Autodesk Inventor part; units mm, degrees
ref_plane "YZ Plane" through (0, 0, 0) normal (1, 0, 0) x (0, 1, 0)
ref_plane "XZ Plane" through (0, 0, 0) normal (0, 1, 0) x (-1, 0, 0)
ref_plane "XY Plane" through (0, 0, 0) normal (0, 0, 1) x (1, 0, 0)
sketch "Sketch1" plane through (0, 0, 0) normal (0, 0, 1) x (1, 0, 0)
  line L0 (0, 0) -> (190, 0)
  line L1 (0, 140) -> (0, 0)
  line L2 (190, 0) -> (190, 30)
  line L3 (190, 30) -> (210, 30)
  line L4 (210, 30) -> (210, 74.5)
  line L5 (186, 140) -> (186, 74.5)
  line L6 (186, 74.5) -> (210, 74.5)
  line L7 (186, 140) -> (0, 140)
  dimension "d2" = 20
  dimension "d3" = 30
  dimension "d4" = 140
  dimension "d49" = 24
  dimension "d50" = 65.5
  dimension "d51" = 210
extrude "Extrusion1" add sketch "Sketch1" along normal blind 3
sketch "Sketch2" plane through (0, 0, 3) normal (0, 0, 1) x (1, 0, 0)
  arc A0 (141.1, 85.2251) -> (158.9, 85.2251) centre (150, 90) ccw
  line L0 (210, 30) -> (210, 74.5)
  line L1 (250, 140) -> (0, 140)
  line L2 (141.1, 94.7749) -> (141.1, 85.2251)
  line L3 (158.9, 94.7749) -> (158.9, 85.2251)
  arc A1 (158.9, 94.7749) -> (141.1, 94.7749) centre (150, 90) ccw
  circle A2 centre (180, 114) radius 6
  line L4 (158.9, 54.7749) -> (158.9, 45.2251)
  arc A3 (158.9, 54.7749) -> (141.1, 54.7749) centre (150, 50) ccw
  line L5 (141.1, 54.7749) -> (141.1, 45.2251)
  arc A4 (141.1, 45.2251) -> (158.9, 45.2251) centre (150, 50) ccw
  arc A5 (101.1, 85.2251) -> (118.9, 85.2251) centre (110, 90) ccw
  arc A6 (118.9, 94.7749) -> (101.1, 94.7749) centre (110, 90) ccw
  line L6 (118.9, 94.7749) -> (118.9, 85.2251)
  line L7 (101.1, 94.7749) -> (101.1, 85.2251)
  arc A7 (63.25, 96.4) -> (76.75, 96.4) centre (70, 100) ccw
  line L8 (63.25, 103.6) -> (63.25, 96.4)
  line L9 (76.75, 103.6) -> (76.75, 96.4)
  arc A8 (76.75, 103.6) -> (63.25, 103.6) centre (70, 100) ccw
  line L10 (76.75, 73.6) -> (76.75, 66.4)
  arc A9 (63.25, 66.4) -> (76.75, 66.4) centre (70, 70) ccw
  line L11 (63.25, 73.6) -> (63.25, 66.4)
  arc A10 (76.75, 73.6) -> (63.25, 73.6) centre (70, 70) ccw
  line L12 (76.75, 43.6) -> (76.75, 36.4)
  arc A11 (63.25, 36.4) -> (76.75, 36.4) centre (70, 40) ccw
  line L13 (63.25, 43.6) -> (63.25, 36.4)
  arc A12 (76.75, 43.6) -> (63.25, 43.6) centre (70, 40) ccw
  line L14 (36.75, 103.6) -> (36.75, 96.4)
  arc A13 (23.25, 96.4) -> (36.75, 96.4) centre (30, 100) ccw
  line L15 (23.25, 103.6) -> (23.25, 96.4)
  arc A14 (36.75, 103.6) -> (23.25, 103.6) centre (30, 100) ccw
  line L16 (36.75, 73.6) -> (36.75, 66.4)
  arc A15 (23.25, 66.4) -> (36.75, 66.4) centre (30, 70) ccw
  line L17 (23.25, 73.6) -> (23.25, 66.4)
  arc A16 (36.75, 73.6) -> (23.25, 73.6) centre (30, 70) ccw
  line L18 (36.75, 43.6) -> (36.75, 36.4)
  arc A17 (23.25, 36.4) -> (36.75, 36.4) centre (30, 40) ccw
  line L19 (23.25, 43.6) -> (23.25, 36.4)
  arc A18 (36.75, 43.6) -> (23.25, 43.6) centre (30, 40) ccw
  circle A19 centre (180, 99) radius 6
  circle A20 centre (180, 84) radius 6
  circle A21 centre (180, 69) radius 6
  point P0 (0, 0)
  dimension "d8" = 60
  dimension "d10" = 17.8
  dimension "d11" = 8.9
  dimension "d12" = 10.1
  dimension "d21" = 12
  dimension "d23" = 30
  dimension "d52" = 26
  dimension "d53" = 50
  dimension "d83" = 40
  dimension "d93" = 40
  dimension "d98" = 40
  dimension "d99" = 40
  dimension "d100" = 13.5
  dimension "d101" = 6.75
  dimension "d102" = 7.65
  dimension "d105" = 30
  dimension "d108" = 40
  dimension "d113" = 15
extrude "Extrusion2" cut sketch "Sketch2" against normal blind 12
sketch "Sketch3" plane through (0, 0, 3) normal (0, 0, 1) x (1, 0, 0)
  circle A0 centre (10, 10) radius 2.75
  circle A1 centre (10, 130) radius 2.75
  circle A2 centre (180, 130) radius 2.75
  circle A3 centre (180, 10) radius 2.75
  circle A4 centre (200, 52) radius 2.75
  line L0 (0, 140) -> (0, 0)
  line L1 (186, 140) -> (0, 140)
  line L2 (0, 0) -> (190, 0)
  line L3 (190, 0) -> (190, 30)
  line L4 (210, 30) -> (210, 74.5)
  line L5 (190, 30) -> (210, 30)
  dimension "d54" = 10
  dimension "d55" = 10
  dimension "d56" = 5.5
  dimension "d57" = 10
  dimension "d58" = 10
  dimension "d59" = 5.5
  dimension "d60" = 10
  dimension "d61" = 10
  dimension "d62" = 5.5
  dimension "d63" = 10
  dimension "d64" = 22
  dimension "d65" = 5.5
  dimension "d67" = 10
  dimension "d68" = 10
  dimension "d69" = 5.5
extrude "Holes" cut sketch "Sketch3" against normal blind 12
sketch "Sketch4" plane through (0, 0, 3) normal (0, 0, 1) x (1, 0, 0)
  line L0 (3, 115) -> (8.2, 115)
  line L1 (8.2, 115) -> (8.2, 104.8)
  line L2 (8.2, 104.8) -> (3, 104.8)
  line L3 (3, 104.8) -> (3, 115)
  line L4 (3, 35.2) -> (8.2, 35.2)
  line L5 (8.2, 35.2) -> (8.2, 25)
  line L6 (8.2, 25) -> (3, 25)
  line L7 (3, 25) -> (3, 35.2)
  line L8 (0, 140) -> (0, 0)
  line L9 (0, 0) -> (190, 0)
  line L10 (186, 140) -> (0, 140)
  dimension "d72" = 3
  dimension "d73" = 3
  dimension "d74" = 25
  dimension "d75" = 25
  dimension "d76" = 10.2
  dimension "d77" = 5.2
  dimension "d78" = 10.2
extrude "Extrusion4" cut sketch "Sketch4" against normal blind 12
equation "\"d45\" = d26"
equation "\"d58\" = d54"
equation "\"d59\" = d56"
equation "\"d60\" = d54"
equation "\"d61\" = d54"
equation "\"d62\" = d56"
equation "\"d63\" = d54"
equation "\"d65\" = d56"
equation "\"d70\" = d26"
equation "\"d79\" = d26"
properties part number "Steckerplatte1"
The model under review builds one solid part; all positions refer to its coordinate system, in mm. A direction names the side the tool comes from. Round coordinates to 2 decimals unless told otherwise and drop trailing zeros. Loops run counter-clockwise (first coordinate to the right, second up) from the corner with the lowest first, then second, coordinate; pieces in that order, holes last. Notation, with made-up numbers: (74, 9.5) -> (94, 9.5) arc R16 ccw to (94, 28.5) -> close; hole circle Ø4 at (59.25, -37.5). An arc over 180 degrees is marked (long way). Answer in a Markdown table with one row per item.
1) Consider section C-C, the plane x = 143.5. Write out the cut boundary in (y, z), plus the area to 3 significant figures.
Taken from the geometry:
| item | result |
|---|---|
| outline | (0, 0) -> (42.27, 0) -> (42.27, 3) -> (0, 3) -> close; (57.73, 0) -> (82.27, 0) -> (82.27, 3) -> (57.73, 3) -> close; (97.73, 0) -> (140, 0) -> (140, 3) -> (97.73, 3) -> close |
| area | 327 mm² |
2) Consider section B-B, the plane x = 180. Write out the cut boundary in (y, z).
Taken from the geometry:
| item | result |
|---|---|
| outline | (0, 0) -> (7.25, 0) -> (7.25, 3) -> (0, 3) -> close; (12.75, 0) -> (63, 0) -> (63, 3) -> (12.75, 3) -> close; (75, 0) -> (78, 0) -> (78, 3) -> (75, 3) -> close; (90, 0) -> (93, 0) -> (93, 3) -> (90, 3) -> close; (105, 0) -> (108, 0) -> (108, 3) -> (105, 3) -> close; (120, 0) -> (127.25, 0) -> (127.25, 3) -> (120, 3) -> close; (132.75, 0) -> (140, 0) -> (140, 3) -> (132.75, 3) -> close |
3) Draft analysis for pull direction Y (two halves, no side actions). For faces 3 (the cylindrical face through (174, 84, 2)), 4 (the cylindrical face through (29.88, 32.35, 1.52)), 5 (the flat face through (104, 71, 3)), state which applies: pulls with the +Y half, pulls with the -Y half, needs draft (parallel to the pull), parting line crosses it, or undercut.
Taken from the geometry:
| item | result |
|---|---|
| face 3 | undercut |
| face 4 | undercut |
| face 5 | needs draft |
4) Wall thickness on line 1 along Y through (x, z) = (10, 2.4); line 2 along X through (y, z) = (36.5, 2.9); line 3 along X through (y, z) = (130, 1.35): over which ranges is each line inside the solid? List them lowest first.
Taken from the geometry:
| item | result |
|---|---|
| line 1 | y = 0 to 7.25, 12.75 to 127.25, 132.75 to 140 |
| line 2 | x = 0 to 23.25, 36.75 to 63.25, 76.75 to 210 |
| line 3 | x = 0 to 7.25, 12.75 to 177.25, 182.75 to 186 |
5) Tool access review of faces 1 (the cylindrical face through (70.12, 77.65, 1.52)), 2 (the flat face through (104, 71, 0)): name each direction out of +Z, -Z, +X, -X, +Y, -Y from which nothing blocks a thin tool from reaching the whole face with its end or side.
Taken from the geometry:
| item | result |
|---|---|
| face 1 | +Z, -Z |
| face 2 | -Z, +X, -X, +Y, -Y |
6) For pin 1 Ø5 at (x, y) = (10, 130) entering from -Z; pin 2 Ø1.5 at (y, z) = (107.5, 1) entering from +X, all flat-tipped, find the tip position at first contact; note any pin that passes through.
Taken from the geometry:
| item | result |
|---|---|
| pin 1 | passes through |
| pin 2 | stops at x = 186 |
7) Consider section A-A, the plane y = 10. Write out the cut boundary in (x, z), plus the area to 3 significant figures.
Taken from the geometry:
| item | result |
|---|---|
| outline | (0, 0) -> (7.25, 0) -> (7.25, 3) -> (0, 3) -> close; (12.75, 0) -> (177.25, 0) -> (177.25, 3) -> (12.75, 3) -> close; (182.75, 0) -> (190, 0) -> (190, 3) -> (182.75, 3) -> close |
| area | 537 mm² |
